from build123d import *

# Parameters (mm, degrees)
SKETCH1_R                       = 85
BOSS_EXTRUDE1_DEPTH             = 25
BOSS_EXTRUDE2_DEPTH             = 10
FILLET1_R                       = 2
SKETCH3_R                       = 9
BOSS_EXTRUDE3_DEPTH             = 6
CUT_EXTRUDE1_DEPTH              = 151.982311708
CUT_EXTRUDE1_DEPTH_BACK         = 157.982311708
CUT_EXTRUDE1_START              = 6
SKETCH4_R                       = 1.55
BOSS_EXTRUDE5_DEPTH             = 9
BOSS_EXTRUDE5_DIRECTION_2_REACH = 158.982
CUT_EXTRUDE9_DEPTH              = 158.386549836
CUT_EXTRUDE9_DEPTH_BACK         = 158.386549836
FILLET3_R                       = 10
FILLET4_R                       = 2
FILLET5_R                       = 2
CUT_EXTRUDE11_DEPTH             = 11


with BuildPart() as part:
    # Sketch1 → Boss-Extrude1 (new body)
    with BuildSketch(Plane(origin=(0, 0, 0), x_dir=(1, 0, 0), z_dir=(0, 1, 0))):
        with Locations(Location((0, 0, 0), (0, 0, 270))):
            Circle(SKETCH1_R)
    extrude(amount=BOSS_EXTRUDE1_DEPTH)

    # Sketch2 → Boss-Extrude2 (add)
    with BuildSketch(Plane.XZ):
        with BuildLine():
            Line((-7.937838503, 79.102722582), (-7.943370347, 72.063533549))
            ThreePointArc((-7.943370347, 72.063533549), (-51.22493832, 51.305513292), (-72.050959732, 8.056624713))
            Line((-72.050959732, 8.056624713), (-79.090148765, 8.062156557))
            ThreePointArc((-79.090148765, 8.062156557), (-56.170794433, 56.259149058), (-7.937838503, 79.102722582))
        make_face()
        with BuildLine():
            Line((-79.102722582, -7.937838503), (-72.063533549, -7.943370347))
            ThreePointArc((-72.063533549, -7.943370347), (-51.305513292, -51.22493832), (-8.056624713, -72.050959732))
            Line((-8.056624713, -72.050959732), (-8.062156557, -79.090148765))
            ThreePointArc((-8.062156557, -79.090148765), (-56.259149058, -56.170794433), (-79.102722582, -7.937838503))
        make_face()
        with BuildLine():
            Line((8.062156557, 79.090148765), (8.056624713, 72.050959732))
            ThreePointArc((8.056624713, 72.050959732), (51.305513292, 51.22493832), (72.063533549, 7.943370347))
            Line((72.063533549, 7.943370347), (79.102722582, 7.937838503))
            ThreePointArc((79.102722582, 7.937838503), (56.259149058, 56.170794433), (8.062156557, 79.090148765))
        make_face()
        with BuildLine():
            Line((72.050959732, -8.056624713), (79.090148765, -8.062156557))
            ThreePointArc((79.090148765, -8.062156557), (56.170794433, -56.259149058), (7.937838503, -79.102722582))
            Line((7.937838503, -79.102722582), (7.943370347, -72.063533549))
            ThreePointArc((7.943370347, -72.063533549), (51.22493832, -51.305513292), (72.050959732, -8.056624713))
        make_face()
    extrude(amount=BOSS_EXTRUDE2_DEPTH)

    # Fillet1
    fillet1_edges = [part.edges().sort_by_distance(p)[0] for p in [
        (79.102722582, -5, 7.937838503),
        (8.062156557, -5, 79.090148765),
        (8.056624713, -5, 72.050959732),
        (72.063533549, -5, 7.943370347),
        (7.937838503, -5, -79.102722582),
        (79.090148765, -5, -8.062156557),
        (72.050959732, -5, -8.056624713),
        (7.943370347, -5, -72.063533549),
        (-79.102722582, -5, -7.937838503),
        (-8.062156557, -5, -79.090148765),
        (-8.056624713, -5, -72.050959732),
        (-72.063533549, -5, -7.943370347),
        (-7.937838503, -5, 79.102722582),
        (-79.090148765, -5, 8.062156557),
        (-72.050959732, -5, 8.056624713),
        (-7.943370347, -5, 72.063533549),
    ]]
    fillet(fillet1_edges, radius=FILLET1_R)

    # Sketch3 → Boss-Extrude3 (add, symmetric)
    with BuildSketch(Plane(origin=(0, 0, 0), x_dir=(0, 0, -1), z_dir=(1, 0, 0))):
        with BuildLine():
            Line((30.34, 25), (-30.34, 25))
            Line((-30.34, 25), (-30.34, 32.86))
            ThreePointArc((-30.34, 32.86), (-29.573250676, 40.170078852), (-27.306377926, 47.161963097))
            Line((-27.306377926, 47.161963097), (-13.792799414, 77.583540747))
            ThreePointArc((-13.792799414, 77.583540747), (31.301699468, 90.103510982), (34.93507351, 43.444513166))
            ThreePointArc((34.93507351, 43.444513166), (31.536487814, 38.51052394), (30.34, 32.64))
            Line((30.34, 32.64), (30.34, 25))
        make_face()
        with Locations((13.908912319, 65.278154724)):
            Circle(SKETCH3_R, mode=Mode.SUBTRACT)
    extrude(amount=BOSS_EXTRUDE3_DEPTH, both=True)

    # Sketch4 → Cut-Extrude1 (cut, two sides: drawn at the far end of the back side and taken through both)
    with BuildSketch(Plane(origin=(6, 0, 0), x_dir=(0, 0, -1), z_dir=(1, 0, 0)).offset(CUT_EXTRUDE1_START - CUT_EXTRUDE1_DEPTH_BACK)):
        with Locations(Location((27.76820523, 71.147141008, 0), (0, 0, 180))):
            Circle(SKETCH4_R)
        with Locations(Location((19.777898603, 79.137447635, 0), (0, 0, 180))):
            Circle(SKETCH4_R)
        with Locations(Location((-6.455762979, 36.923172798, 0), (0, 0, 180))):
            Circle(SKETCH4_R)
        with Locations(Location((-14.446069607, 44.913479426, 0), (0, 0, 180))):
            Circle(SKETCH4_R)
    extrude(amount=CUT_EXTRUDE1_DEPTH + CUT_EXTRUDE1_DEPTH_BACK, mode=Mode.SUBTRACT)

    # Sketch7 → Boss-Extrude5 (add)
    with BuildSketch(Plane(origin=(6, 0, 0), x_dir=(0, 0, -1), z_dir=(1, 0, 0))):
        with BuildLine():
            Line((36.34, 25), (36.34, 32.64))
            ThreePointArc((36.34, 32.64), (37.057892688, 36.162314364), (39.097044106, 39.122707899))
            ThreePointArc((39.097044106, 39.122707899), (34.744470977, 95.01750369), (-19.276145073, 80.019299435))
            Line((-19.276145073, 80.019299435), (-32.789723585, 49.597721785))
            ThreePointArc((-32.789723585, 49.597721785), (-35.442666062, 41.415053962), (-36.34, 32.86))
            Line((-36.34, 32.86), (-36.34, 25))
            Line((-36.34, 25), (-27.34, 25))
            ThreePointArc((-27.34, 25), (-22.752054714, 51.854864954), (-13.792799414, 77.583540747))
            ThreePointArc((-13.792799414, 77.583540747), (31.301699468, 90.103510982), (34.93507351, 43.444513166))
            ThreePointArc((34.93507351, 43.444513166), (31.536487814, 38.51052394), (30.34, 32.64))
            Line((30.34, 32.64), (30.34, 25))
            Line((30.34, 25), (36.34, 25))
        make_face()
    extrude(amount=BOSS_EXTRUDE5_DEPTH)

    # Boss-Extrude5 direction 2: up to this face of the body (flat: up to its plane)
    boss_extrude5_direction_2_end = Plane(part.part.faces().sort_by_distance((-6, 56.749631144, -7.806138982))[0])
    # Sketch7 → Boss-Extrude5 direction 2 (add, up to the picked face)
    with BuildSketch(Plane(origin=(6, 0, 0), x_dir=(0, 0, -1), z_dir=(1, 0, 0)), mode=Mode.PRIVATE) as boss_extrude5_direction_2_sk1:
        with BuildLine():
            Line((36.34, 25), (36.34, 32.64))
            ThreePointArc((36.34, 32.64), (37.057892688, 36.162314364), (39.097044106, 39.122707899))
            ThreePointArc((39.097044106, 39.122707899), (34.744470977, 95.01750369), (-19.276145073, 80.019299435))
            Line((-19.276145073, 80.019299435), (-32.789723585, 49.597721785))
            ThreePointArc((-32.789723585, 49.597721785), (-35.442666062, 41.415053962), (-36.34, 32.86))
            Line((-36.34, 32.86), (-36.34, 25))
            Line((-36.34, 25), (-27.34, 25))
            ThreePointArc((-27.34, 25), (-22.752054714, 51.854864954), (-13.792799414, 77.583540747))
            ThreePointArc((-13.792799414, 77.583540747), (31.301699468, 90.103510982), (34.93507351, 43.444513166))
            ThreePointArc((34.93507351, 43.444513166), (31.536487814, 38.51052394), (30.34, 32.64))
            Line((30.34, 32.64), (30.34, 25))
            Line((30.34, 25), (36.34, 25))
        make_face()
    boss_extrude5_direction_2_tool1 = split(extrude(boss_extrude5_direction_2_sk1.sketch, amount=-BOSS_EXTRUDE5_DIRECTION_2_REACH, mode=Mode.PRIVATE), bisect_by=boss_extrude5_direction_2_end, keep=Keep.BOTH, mode=Mode.PRIVATE)
    add(boss_extrude5_direction_2_tool1.solids().sort_by(Axis((6, 91.050112, -31.964893), (-1, 0, 0)))[0])

    # Sketch8 → Cut-Extrude9 (cut, two sides: drawn at the far end of the back side and taken through both)
    with BuildSketch(Plane.XY.offset(-CUT_EXTRUDE9_DEPTH_BACK)):
        with BuildLine():
            Line((15, 101.589990006), (9, 101.589990006))
            ThreePointArc((9, 101.589990006), (10.277543258, 63.189256484), (14.5, 25))
            Line((14.5, 25), (15, 25))
            Line((15, 25), (15, 101.589990006))
        make_face()
    extrude(amount=CUT_EXTRUDE9_DEPTH + CUT_EXTRUDE9_DEPTH_BACK, mode=Mode.SUBTRACT)

    # Fillet3
    fillet3_edges = [part.edges().sort_by_distance(p)[0] for p in [
        (-6, 28.82, -36.34),
        (-6, 36.162314364, -37.057892688),
        (-6, 95.01750369, -34.744470977),
        (-6, 64.80851061, 26.032934329),
        (-6, 41.415053962, 35.442666062),
        (-6, 28.93, 36.34),
    ]]
    fillet(fillet3_edges, radius=FILLET3_R)

    # Fillet4
    fillet4_edges = [part.edges().sort_by_distance(p)[0] for p in [
        (9.25, 25, -36.34),
        (-6, 25, 0),
        (9.25, 25, 36.34),
        (-3.071067812, 25, -33.411067812),
        (-3.071067812, 25, 33.411067812),
    ]]
    fillet(fillet4_edges, radius=FILLET4_R)

    # Fillet5
    fillet5_edges = [part.edges().sort_by_distance(p)[0] for p in [
        (14.5, 25, -34.34),
        (14.5, 25, 32.84),
    ]]
    fillet(fillet5_edges, radius=FILLET5_R)

    # Sketch4<3> → Cut-Extrude11 (cut)
    with BuildSketch(Plane(origin=(6, 0, 0), x_dir=(0, 0, -1), z_dir=(1, 0, 0))):
        Polygon((-0.41, 36.11), (28.581378029, 65.101378029), (13.732135624, 79.950620434), (-15.259242405, 50.959242405), align=None)
    extrude(amount=-CUT_EXTRUDE11_DEPTH, mode=Mode.SUBTRACT)


solid = part.part
Work out the finished part from the listing and answer in its coordinate system (mm). A direction names the side the tool comes from. Round coordinates to 2 decimals unless told otherwise and drop trailing zeros. Write each loop counter-clockwise with the first axis right and the second up, starting at its lowest first coordinate (ties: lowest second). Pieces come first, ordered by that corner, then holes.
1) A cutting plane is placed at B-B (z = 50). Give the vertices of the cut face in (x, y).
2) A cutting plane is placed at A-A (x = 28). Give the vertices of the cut face in (y, z), plus the area to 3 significant figures.
3) Given pin 1 Ø3 at (x, y) = (7, 29.5) entering from +Z; pin 2 Ø3.5 at (y, z) = (79.14, -19.78) entering from -X; pin 3 Ø1.5 at (x, z) = (16, 1.5) entering from -Y; pin 4 Ø2.5 at (y, z) = (71.15, -27.77) entering from -X, each flat-ended and moving along its own axis, determine where each tip first touches the part or whether it passes through.
4) A tool of negligible diameter and unlimited length cuts with its end or side. For faces 5 (the cylindrical face through (7.65, 82.2, -39.06)), 6 (the flat face through (9, 30, 36.34)), 7 (the cylindrical face through (-56.685, -4.93, 55.741)), from which of +Z, -Z, +X, -X, +Y, -Y can it reach the whole face along a straight path? Write none if from no direction.
5) The mould has two halves that part along Z. Classify faces 1 (the flat face through (0.58, 72.42, -21.26)), 2 (the cylindrical face through (-51.77, -4.93, -50.755)), 3 (the cylindrical face through (-51.721, 12.325, -67.453)), 4 (the cylindrical face through (-55.741, -4.93, -56.685)): pulls with the +Z half, pulls with the -Z half, needs draft (parallel to the pull), parting line crosses it, or undercut.
6) A cutting plane is placed at C-C (x = 0). Give the number of separate pieces and of enclosed holes in the cut face, plus the area to 3 significant figures.
7) Straight lines are drawn through the part: line 1 (X direction, y = 37, z = 19); line 2 (Y direction, x = 18.5, z = 1.5); line 3 (Y direction, x = -36, z = -64). For each, find the intervals that lie inside material, in ascending order.
Completed:
1. outline: (-68.74, 0) - (-61.81, 0) - (-61.81, -10) - (-52.5, -10) - (-52.5, 0) - (52.5, 0) - (52.5, -10) - (61.81, -10) - (61.81, 0) - (68.74, 0) - (68.74, 25) - (-68.74, 25) - close
2. outline: (-10, -74.41) - (0, -74.41) - (0, -80.26) - (25, -80.26) - (25, 80.26) - (0, 80.26) - (0, 74.41) - (-10, 74.41) - (-10, 66.87) - (0, 66.87) - (0, -66.87) - (-10, -66.87) - close
2. area: 4,160 mm2
3. pin 1: stops at z = 36.34
3. pin 2: stops at x = -6
3. pin 3: stops at y = 0
3. pin 4: passes through
4. face 5: +X
4. face 6: +Z, +X, -X, +Y
4. face 7: +Z, -X, -Y
5. face 1: undercut
5. face 2: undercut
5. face 3: parting line crosses it
5. face 4: pulls with the -Z half
6. separate pieces: 1
6. enclosed holes: 5
6. area: 8,360 mm2
7. line 1: x = -6 to 6
7. line 2: y = 0 to 25
7. line 3: y = -10 to 25
